Geometry check sheet. Reference: the model listing, model coordinates, mm. Face numbers are marked on the shaded views. A direction names the side the tool comes from. Coordinates: 2 decimals unless noted, no trailing zeros. Loops run counter-clockwise (first coordinate to the right, second up) from the corner with the lowest first, then second, coordinate; pieces in that order, holes last. Notation, with made-up numbers: M 60,24.25 L 64,24.25 A25 ccw 64,37.25 Z; hole C 85.5,55.25 d11. An arc over 180 degrees is marked long. Use CSV: the item, a comma, the result in double quotes.
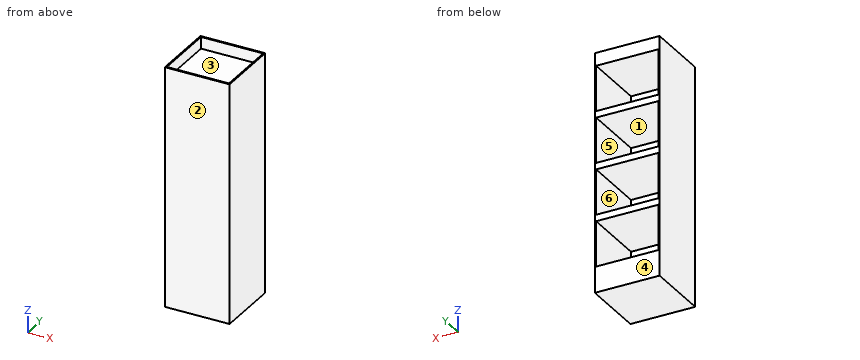
```python
from build123d import *

# Parameters (mm, degrees)
F0_W     = 500
F0_H     = 500
F1_DEPTH = 1850
F2_W     = 480
F2_H     = 350
F3_DEPTH = 490
F4_W     = 480
F4_H     = 480
F5_DEPTH = 90


with BuildPart() as f1:
    # F0 (on Top) → F1 (new body)
    with BuildSketch(Plane.XY):
        with Locations((-250, 250)):
            Rectangle(F0_W, F0_H)
    extrude(amount=F1_DEPTH)

    # F2 (on face) → F3 (cut)
    with BuildSketch(Plane(origin=(0, 500, 0), x_dir=(-1, 0, 0), z_dir=(0, 1, 0))):
        with Locations((250, 1575)):
            Rectangle(F2_W, F2_H)
        with Locations((250, 1175)):
            Rectangle(F2_W, F2_H)
        with Locations((250, 775)):
            Rectangle(F2_W, F2_H)
        with Locations((250, 375)):
            Rectangle(F2_W, F2_H)
    extrude(amount=-F3_DEPTH, mode=Mode.SUBTRACT)

    # F4 (on face) → F5 (cut)
    with BuildSketch(Plane.XY.offset(1850)):
        with Locations((-250, 250)):
            Rectangle(F4_W, F4_H)
    extrude(amount=-F5_DEPTH, mode=Mode.SUBTRACT)


solid = f1.part
```
1. Set-up check for the marked faces 1 and 2: record each of +Z, -Z, +X, -X, +Y, -Y from which the full face is reachable in a straight line by a thin tool's end or side.
The answers:
face 1,"+Y"
face 2,"+Z, -Z, +X, -X, -Y"
2. Thickness scan on line 1 (Z direction, x = -226, y = 256); line 2 (X direction, y = 110, z = 1409); line 3 (Y direction, x = -272, z = 467.5). Record the ranges inside material, lowest first. Write a range as [from, to].
The answers:
line 1,"[0, 200], [550, 600], [950, 1000], [1350, 1400], [1750, 1760]"
line 2,"[-500, -490], [-10, 0]"
line 3,"[0, 10]"
3. Section check A-A, the plane x = -159. Record the cut outline in (y, z).
The answers:
outline,"M 0,0 L 500,0 L 500,200 L 10,200 L 10,550 L 500,550 L 500,600 L 10,600 L 10,950 L 500,950 L 500,1000 L 10,1000 L 10,1350 L 500,1350 L 500,1400 L 10,1400 L 10,1750 L 500,1750 L 500,1850 L 490,1850 L 490,1760 L 10,1760 L 10,1850 L 0,1850 Z"
4. Section check B-B, the plane y = 84. Record the cut outline in (x, z).
The answers:
outline,"M -500,0 L 0,0 L 0,1850 L -10,1850 L -10,1760 L -490,1760 L -490,1850 L -500,1850 Z; hole M -490,200 L -10,200 L -10,550 L -490,550 Z; hole M -490,600 L -10,600 L -10,950 L -490,950 Z; hole M -490,1000 L -10,1000 L -10,1350 L -490,1350 Z; hole M -490,1400 L -10,1400 L -10,1750 L -490,1750 Z"
5. Section check C-C, the plane z = 869. Record the cut outline in (x, y), plus the area to 3 significant figures.
The answers:
outline,"M -500,0 L 0,0 L 0,500 L -10,500 L -10,10 L -490,10 L -490,500 L -500,500 Z"
area,"14,800 mm^2"
6. Gauge pin test, flat ends, axial feed: P1, Ø3, axis at x = -235.5, y = 361, coming from the +Z side; P2, Ø8, axis at y = 62, z = 1039, coming from the +X side. Record the tip position at first contact, or that the pin passes through.
The answers:
P1,"z = 1760"
P2,"x = 0"
7. Release check for a two-part mould opening along Z. For the marked faces 3, 4, 5 and 6 record: +Z half, -Z half, draft (parallel to the pull), parting line (faces both ways), or undercut.
The answers:
face 3,"+Z half"
face 4,"draft"
face 5,"undercut"
face 6,"undercut"
